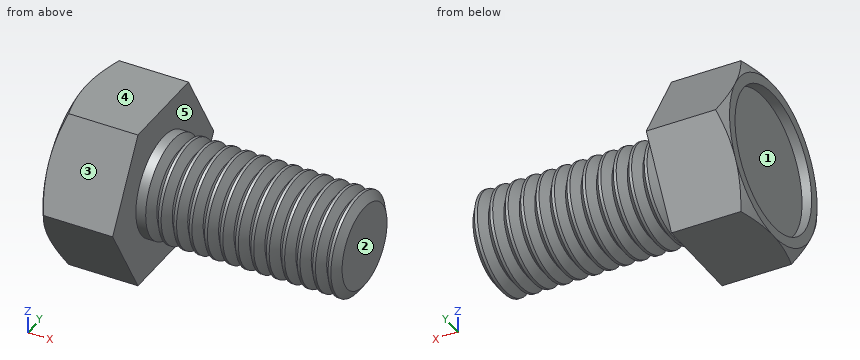
```python
from build123d import *

# Parameters (mm, degrees)
SKETCH2_R       = 4.665127021
HEX_DIE_DEPTH   = 3.8
SKETCH4_R       = 3.5
INDENT_DEPTH    = 0.475
THDSCHPAT_COUNT = 13
THDSCHPAT_PITCH = 0.766666667


with BuildPart() as part:
    # BodySke → Base-Revolve (revolve)
    with BuildSketch(Plane.XY, mode=Mode.PRIVATE) as base_revolve_sk:
        Polygon((3.8, 2.5), (3.8, 4.618937644), (0.357343816, 4.618937644), (0, 4), (0, 0), (13.8, 0), (13.8, 2.5), align=None)
    revolve(base_revolve_sk.sketch.rotate(Axis((-25.4, 0, 0), (1, 0, 0)), 90), axis=Axis((-25.4, 0, 0), (1, 0, 0)))

    # Sketch2 → Hex-Die (cut)
    with BuildSketch(Plane(origin=(0, 0, 0), x_dir=(0, 0, -1), z_dir=(1, 0, 0))):
        Circle(SKETCH2_R)
        Polygon((-4, 2.309401087), (0, 4.618802174), (4, 2.309401087), (4, -2.309401087), (0, -4.618802174), (-4, -2.309401087), align=None, mode=Mode.SUBTRACT)
    extrude(amount=HEX_DIE_DEPTH, mode=Mode.SUBTRACT)

    # Sketch4 → Indent (cut)
    with BuildSketch(Plane(origin=(0, 0, 0), x_dir=(0, 0, -1), z_dir=(1, 0, 0))):
        with Locations(Location((0, 0, 0), (0, 0, 180))):
            Circle(SKETCH4_R)
    extrude(amount=INDENT_DEPTH, mode=Mode.SUBTRACT)

    # ThdSchSke → ThreadSchematic (revolve, cut)
    with BuildSketch(Plane.XY):
        Polygon((4.6, -2.055), (4.288407645, -2.5), (4.288407645, -3.125), (4.911592355, -3.125), (4.911592355, -2.5), align=None)
    threadschematic = revolve(axis=Axis((-3.175, 0, 0), (1, 0, 0)), mode=Mode.SUBTRACT)

    # ThdSchPat: ThreadSchematic ×13
    with Locations(*[(i * THDSCHPAT_PITCH, 0, 0) for i in range(1, THDSCHPAT_COUNT)]):
        add(threadschematic, mode=Mode.SUBTRACT)


solid = part.part
```
Work out the finished part from the listing and answer in its coordinate system (mm). Face numbers are marked on the shaded views. A direction names the side the tool comes from. Give positions to 0.01 mm unless a question says otherwise; leave off trailing zeros. Loops run counter-clockwise (first coordinate to the right, second up) from the corner with the lowest first, then second, coordinate; pieces in that order, holes last. Notation, with made-up numbers: (-34, 10.5) - (-2, 10.5) arc R37 ccw to (-2, 46.5) - close; hole circle Ø4 at (-23, 73.5). An arc over 180 degrees is marked (long way). Use CSV: the item, a comma, the result in double quotes. Start each with the question number.
(1) Find section A-A, the plane x = 2.75. Determine the outline of the cut face in (y, z).
(2) Find the intervals of material crossed by L1, parallel to X at y = 0, z = 1.5 (3 decimals); L2, parallel to Y at x = 0.3, z = 0; L3, parallel to X at y = 2, z = -2.5 (3 decimals), in increasing order.
(3) Determine the mould class of the marked faces 1, 2 and 3 for opening direction Y: released by +Y, released by -Y, zero draft, split by the parting line, or undercut.
(4) Each of these flat-tipped pins is pushed along its axis until it touches: pin 1 (3 mm diameter, centred on x = 11, y = 2.5, fed in from +Z); pin 2 (1.5 mm diameter, centred on x = 8, z = 2.5, fed in from -Y); pin 3 (3.5 mm diameter, centred on y = 0.5, z = -0.5, fed in from -X) (3 decimals). Where does it stop, or does it pass through?
(5) A tool of negligible diameter and unlimited length cuts with its end or side. For the marked faces 4 and 5, from which of +Z, -Z, +X, -X, +Y, -Y can it reach the whole face along a straight path? Write none if from no direction.
Results found:
1,outline,"(-4.62, 0) - (-2.31, -4) - (2.31, -4) - (4.62, 0) - (2.31, 4) - (-2.31, 4) - close"
2,L1,"0.475 to 13.8"
2,L2,"-4.52 to -3.5, 3.5 to 4.52"
2,L3,"0.475 to 3.8"
3,face 1,"undercut"
3,face 2,"zero draft"
3,face 3,"released by -Y"
4,pin 1,"z = 2.29"
4,pin 2,"y = -1.79"
4,pin 3,"x = 0.475"
5,face 4,"+Z, +X, -X, +Y, -Y"
5,face 5,"+X"
